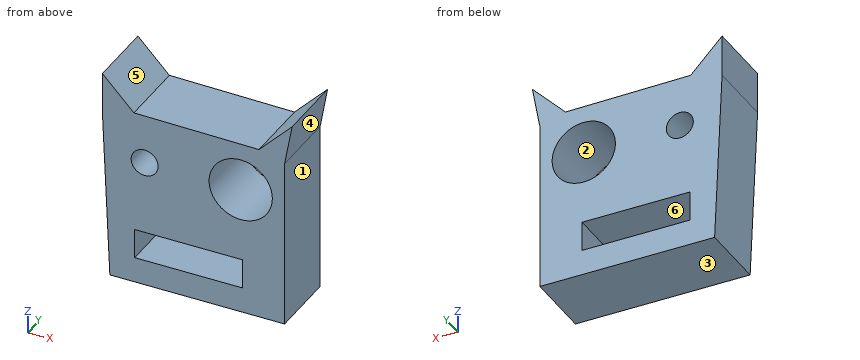
from build123d import *

# Parameters (mm, degrees)
F0_R     = 4.971253
F0_R_2   = 11.668616
F1_DEPTH = 25.4


with BuildPart() as f1:
    # F0 (on Front) → F1 (new body)
    with BuildSketch(Plane.XZ):
        Polygon((19.697119, 37.714638), (-26.415516, 38.325403), (-38.020018, 50.235286), (-38.020018, 34.966201), (-35.271585, -27.637042), (29.163949, -27.637042), (29.163949, 34.966201), (31.912383, 50.235286), align=None)
        Polygon((-26.110133, -12.67334), (-26.110133, -7.17647), (-21.224027, -7.17647), (-16.33792, -7.17647), (-12.062577, -7.17647), (-6.260324, -7.17647), (-2.901126, -7.17647), (2.290364, -7.17647), (6.260325, -7.17647), (9.314141, -7.17647), (13.589485, -7.17647), (13.589485, -12.67334), (13.589485, -18.17021), (9.314141, -18.17021), (6.260325, -18.17021), (2.290364, -18.17021), (-2.901126, -18.17021), (-6.260324, -18.17021), (-12.062577, -18.17021), (-16.33792, -18.17021), (-21.224027, -18.17021), (-26.110133, -18.17021), align=None, mode=Mode.SUBTRACT)
        with Locations((-22.445554, 20.002501)):
            Circle(F0_R, mode=Mode.SUBTRACT)
        with Locations((12.97872, 20.002501)):
            Circle(F0_R_2, mode=Mode.SUBTRACT)
    extrude(amount=F1_DEPTH)


solid = f1.part
Part model, mm, in its own coordinate system. Face numbers are marked on the shaded views. A direction names the side the tool comes from. Give positions to 0.01 mm unless a question says otherwise; leave off trailing zeros. Write each loop counter-clockwise with the first axis right and the second up, starting at its lowest first coordinate (ties: lowest second). Pieces come first, ordered by that corner, then holes.
1) Probe L1, parallel to Z at x = -22, y = -5.5; L2, parallel to X at y = -20.5, z = -11.5; L3, parallel to X at y = -4.75, z = 24. List the from-to ranges inside material, lowest first.
Resolved:
L1: z = -27.64 to -18.17, -7.18 to 15.05, 24.95 to 38.27
L2: x = -35.98 to -26.11, 13.59 to 29.16
L3: x = -37.54 to -25.4, -19.49 to 2.02, 23.94 to 29.16
2) Cut at B-B on y = -2. Write the cut outline in (x, z).
Resolved:
outline: (-38.02, 34.97) - (-35.27, -27.64) - (29.16, -27.64) - (29.16, 34.97) - (31.91, 50.24) - (19.7, 37.71) - (-26.42, 38.33) - (-38.02, 50.24) - close; hole circle Ø9.94 at (-22.45, 20); hole (-26.11, -18.17) - (13.59, -18.17) - (13.59, -7.18) - (-26.11, -7.18) - close; hole circle Ø23.34 at (12.98, 20)
3) Cut at A-A on z = -9. Write the cut outline in (x, y), then the cut area to 3 significant figures.
Resolved:
outline: (-36.09, -25.4) - (-26.11, -25.4) - (-26.11, 0) - (-36.09, 0) - close; (13.59, -25.4) - (29.16, -25.4) - (29.16, 0) - (13.59, 0) - close
area: 649 mm2
4) Two-plate mould, pull along Z, no slides. Class the marked faces 1, 2 and 3: released by +Z, released by -Z, zero draft, split by the parting line, or undercut.
Resolved:
face 1: zero draft
face 2: undercut
face 3: released by -Z
5) Which spindle directions (+Z, -Z, +X, -X, +Y, -Y) get a long thin tool onto all of the face, cutting with end or side? Do the marked faces 4, 5 and 6. Say none if no direction does.
Resolved:
face 4: -Z, +X, +Y, -Y
face 5: +Z, +Y, -Y
face 6: +Y, -Y
6) Cut at C-C on x = -21.5. Write the cut outline in (y, z).
Resolved:
outline: (-25.4, -27.64) - (0, -27.64) - (0, -18.17) - (-25.4, -18.17) - close; (-25.4, -7.18) - (0, -7.18) - (0, 15.12) - (-25.4, 15.12) - close; (-25.4, 24.88) - (0, 24.88) - (0, 38.26) - (-25.4, 38.26) - close
7) Pin check, flat tips, straight feed: pin 1 (5 mm diameter, centred on y = -21.5, z = 12.5, fed in from +X); pin 2 (8 mm diameter, centred on x = -16.5, y = -12.5, fed in from +Z); pin 3 (4 mm diameter, centred on x = 22, y = -6.5, fed in from +Z). Stop position of each tip, or through.
Resolved:
pin 1: stops at x = 29.16
pin 2: stops at z = 38.25
pin 3: stops at z = 42.13
8) Cut at D-D on z = 39.5. Write the cut outline in (x, y), then the cut area to 3 significant figures.
Resolved:
outline: (-38.02, -25.4) - (-27.56, -25.4) - (-27.56, 0) - (-38.02, 0) - close; (21.44, -25.4) - (29.98, -25.4) - (29.98, 0) - (21.44, 0) - close
area: 483 mm2
